from build123d import *

# Parameters (mm, degrees)
F1_DEPTH = 50.8
F2_W     = 50.8
F2_H     = 127
F3_DEPTH = 50.8
F4_W     = 50.8
F4_H     = 25.4
F5_DEPTH = 25.4
F6_W     = 50.8
F6_H     = 25.4
F7_DEPTH = 25.4


with BuildPart() as f1:
    # F0 (on Top) → F1 (new body)
    with BuildSketch(Plane.XY):
        Polygon((83.328486, 79.250188), (-119.871514, 79.250188), (-119.871514, -47.749812), (83.328486, -47.749812), (83.328486, -9.649812), (-18.271514, -9.649812), (-18.271514, 41.150188), (83.328486, 41.150188), align=None)
    extrude(amount=F1_DEPTH)

    # F2 (on face) → F3 (join)
    with BuildSketch(Plane.XY.offset(50.8)):
        with Locations((-94.471514, 15.750188)):
            Rectangle(F2_W, F2_H)
    extrude(amount=F3_DEPTH)

    # F4 (on face) → F5 (join)
    with BuildSketch(Plane.XY.offset(101.6)):
        with Locations((-94.471514, -35.049812)):
            Rectangle(F4_W, F4_H)
    extrude(amount=F5_DEPTH)

    # F6 (on face) → F7 (join)
    with BuildSketch(Plane.XY.offset(101.6)):
        with Locations((-94.471514, 66.550188)):
            Rectangle(F6_W, F6_H)
    extrude(amount=F7_DEPTH)


solid = f1.part
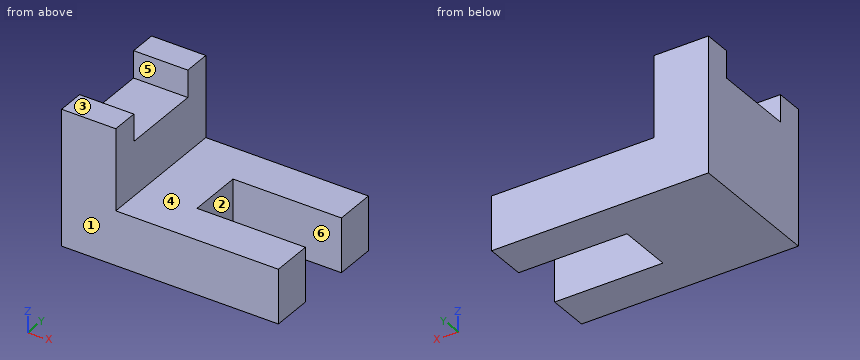
Here's how the part is built. I have some questions about the finished solid (model axes, mm). Face numbers are marked on the shaded views. A direction names the side the tool comes from. Coordinates: 2 decimals unless noted, no trailing zeros. Write each loop counter-clockwise with the first axis right and the second up, starting at its lowest first coordinate (ties: lowest second). Pieces come first, ordered by that corner, then holes.
1) I'm going to push flat-ended pins straight in: pin 1 (6 mm diameter, centred on y = 27.5, z = 74, fed in from +X); pin 2 (3 mm diameter, centred on y = 30.5, z = 35, fed in from +X). Where does each tip first touch, or does it pass through?
Filled in:
pin 1: stops at x = -69.07
pin 2: stops at x = -18.27
2) If we section it at A-A (x = 25.5): List the corners of the cut face in (y, z) for me, plus the area to 3 significant figures.
Filled in:
outline: (-47.75, 0) - (-9.65, 0) - (-9.65, 50.8) - (-47.75, 50.8) - close; (41.15, 0) - (79.25, 0) - (79.25, 50.8) - (41.15, 50.8) - close
area: 3,870 mm2
3) If we section it at D-D (y = -33.5): List the corners of the cut face in (x, z) for me, plus the area to 3 significant figures.
Filled in:
outline: (-119.87, 0) - (83.33, 0) - (83.33, 50.8) - (-69.07, 50.8) - (-69.07, 127) - (-119.87, 127) - close
area: 14,200 mm2
4) If I drill on line 1 (Y direction, x = 45.5, z = 7); line 2 (Z direction, x = -27.5, y = -5.5); line 3 (X direction, y = 41.5, z = 97), over which ranges is the centre line in solid material (lowest first)?
Filled in:
line 1: y = -47.75 to -9.65, 41.15 to 79.25
line 2: z = 0 to 50.8
line 3: x = -119.87 to -69.07
5) If we section it at C-C (z = 46.5): List the corners of the cut face in (x, y) for me.
Filled in:
outline: (-119.87, -47.75) - (83.33, -47.75) - (83.33, -9.65) - (-18.27, -9.65) - (-18.27, 41.15) - (83.33, 41.15) - (83.33, 79.25) - (-119.87, 79.25) - close
6) If we section it at B-B (z = 115): List the corners of the cut face in (x, y) for me.
Filled in:
outline: (-119.87, -47.75) - (-69.07, -47.75) - (-69.07, -22.35) - (-119.87, -22.35) - close; (-119.87, 53.85) - (-69.07, 53.85) - (-69.07, 79.25) - (-119.87, 79.25) - close
7) Which directions (+Z, -Z, +X, -X, +Y, -Y) give clear straight access to the entire face, cutting with the end or side of a thin tool? Please do the marked faces 4, 5 and 6.
Filled in:
face 4: +Z, +X, +Y, -Y
face 5: +Z, +X, -X
face 6: +Z, -Z, +X
8) Thinking about a two-plate mould opening in Y: for the marked faces 1, 2 and 3, which applies, +Y half, -Y half, draft (parallel to the pull), parting line (faces both ways), or undercut?
Filled in:
face 1: -Y half
face 2: undercut
face 3: draft
